from build123d import *

# Parameters (mm, degrees)
BOSS_EXTRUDE1_DEPTH = 4
BOSS_EXTRUDE2_DEPTH = 2.5
CHAMFER1_SIZE       = 1
SKETCH4_W           = 6
SKETCH4_H           = 1.5
CUT_EXTRUDE1_DEPTH  = 2.0001
CHAMFER2_SIZE       = 1
SKETCH5_W           = 39.95
SKETCH5_H           = 3.0001
BOSS_EXTRUDE3_DEPTH = 7.1


with BuildPart() as part:
    # Sketch2 → Boss-Extrude1 (new body)
    with BuildSketch(Plane.XY):
        Polygon((-29.9999, -3.0001), (29.9999, -3.0001), (29.9999, -34.771531454), (23.171531454, -41.5999), (-23.171531454, -41.5999), (-29.9999, -34.771531454), align=None)
        Polygon((-28, -33.943145751), (-28, -5), (28, -5), (28, -33.943145751), (22.343145751, -39.6), (-22.343145751, -39.6), align=None, mode=Mode.SUBTRACT)
    extrude(amount=-BOSS_EXTRUDE1_DEPTH)

    # Sketch3 → Boss-Extrude2 (add)
    with BuildSketch(Plane.XY):
        Polygon((-32, 0), (32, 0), (32, -35.6), (24, -43.6), (-24, -43.6), (-32, -35.6), align=None)
    extrude(amount=BOSS_EXTRUDE2_DEPTH)

    # Chamfer1
    chamfer1_edges = [part.edges().sort_by_distance(p)[0] for p in [
        (-32, -17.8, 2.5),
        (-28, -39.6, 2.5),
        (0, -43.6, 2.5),
        (28, -39.6, 2.5),
        (32, -17.8, 2.5),
        (0, 0, 2.5),
    ]]
    chamfer(chamfer1_edges, length=CHAMFER1_SIZE)

    # Sketch4 → Cut-Extrude1 (cut)
    with BuildSketch(Plane.XZ.offset(43.6)):
        Rectangle(SKETCH4_W, SKETCH4_H)
    extrude(amount=-CUT_EXTRUDE1_DEPTH, mode=Mode.SUBTRACT)

    # Chamfer2
    # the kernel refuses this chamfer: 1 mm, written as the material it adds along each edge
    with BuildSketch(Plane(origin=(3, -43.6, 0.75), x_dir=(0.027495876610586487, 0, -0.9996219169112968), z_dir=(0, 1, 0))) as chamfer2_piece_1_section:
        Polygon((CHAMFER2_SIZE * 0.999621916911, CHAMFER2_SIZE * 0.0274958766106), (-CHAMFER2_SIZE * 0.0274958766106, CHAMFER2_SIZE * 0.999621916911), (0, 0), align=None)
    chamfer2_piece_1 = extrude(amount=4.571782988, mode=Mode.PRIVATE)
    chamfer2_piece_1 = split(chamfer2_piece_1, bisect_by=Plane(origin=(2.65, -42.59995, 0), z_dir=(0, 0, 1)), keep=Keep.TOP, mode=Mode.PRIVATE)
    add(chamfer2_piece_1)
    with BuildSketch(Plane(origin=(-3, -43.6, 0.75), x_dir=(-0.027495876610586487, 0, -0.9996219169112968), z_dir=(0, 1, 0))) as chamfer2_piece_2_section:
        Polygon((CHAMFER2_SIZE * 0.999621916911, -CHAMFER2_SIZE * 0.0274958766106), (-CHAMFER2_SIZE * 0.0274958766106, -CHAMFER2_SIZE * 0.999621916911), (0, 0), align=None)
    chamfer2_piece_2 = extrude(amount=4.571782988, mode=Mode.PRIVATE)
    chamfer2_piece_2 = split(chamfer2_piece_2, bisect_by=Plane(origin=(-2.65, -42.59995, 0), z_dir=(0, 0, 1)), keep=Keep.TOP, mode=Mode.PRIVATE)
    add(chamfer2_piece_2)

    # Sketch5 → Boss-Extrude3 (add)
    with BuildSketch(Plane(origin=(0, 0, 0), x_dir=(-1, 0, 0), z_dir=(0, 0, -1))):
        with Locations((0, -1.50005)):
            Rectangle(SKETCH5_W, SKETCH5_H)
    extrude(amount=BOSS_EXTRUDE3_DEPTH)


solid = part.part
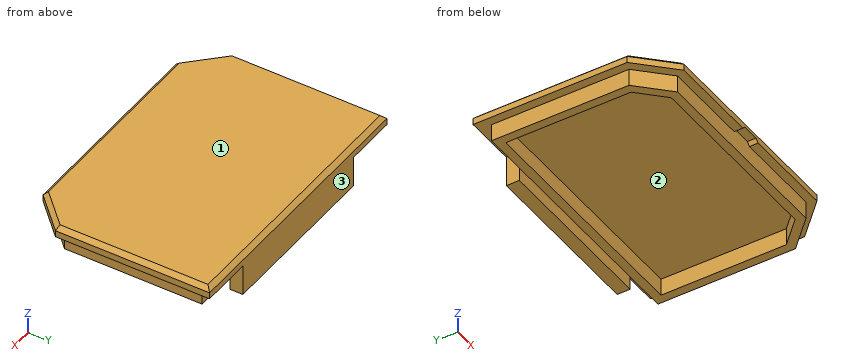
Geometry check sheet. Reference: the model listing, model coordinates, mm. Face numbers are marked on the shaded views. Coordinates: 2 decimals unless noted, no trailing zeros. Order: outer loops, then holes, each group sorted by start corner. A loop starts at its lowest first (then second) coordinate and runs counter-clockwise, first axis right, second up. Notation, with made-up numbers: (29, 45) - (80, 45) arc R6 cw to (80, 51) - close; hole circle Ø2 at (15, 33.5). An arc over 180 degrees is marked (long way). Answer in a Markdown table with one row per item. Add a question column.
1) Release check for a two-part mould opening along Y. For the marked faces 1, 2 and 3 record: +Y half, -Y half, draft (parallel to the pull), parting line (faces both ways), or undercut.
2) Cross-section at B-B, the plane x = 21.5. Record the cut outline in (y, z), then the cut area to 3 significant figures.
3) Gauge pin test, flat ends, axial feed: P1, Ø1.2, axis at x = -4, z = -2, coming from the -Y side; P2, Ø6, axis at x = 7.5, y = -31.5, coming from the -Z side; P3, Ø2, axis at y = -26, z = -1.5, coming from the -X side. Record the tip position at first contact, or that the pin passes through.
4) Cross-section at A-A, the plane y = -6.5. Record the cut outline in (x, z).
5) Material ranges on line 1 along X through (y, z) = (-19, -2); line 2 along Y through (x, z) = (-10, -3.75); line 3 along Z through (x, y) = (-26, -23.5), recorded low to high. Write a range as [from, to].
6) Cross-section at C-C, the plane z = -5.75. Record the cut outline in (x, y) (3 decimals), then the cut area to 3 significant figures.
Check result:
| question | item | result |
|---|---|---|
| 1 | face 1 | draft |
| 1 | face 2 | undercut |
| 1 | face 3 | +Y half |
| 2 | outline | (-43.6, 0) - (-41.6, 0) - (-41.6, -4) - (-39.6, -4) - (-39.6, 0) - (-5, 0) - (-5, -4) - (-3, -4) - (-3, 0) - (0, 0) - (0, 1.5) - (-1, 2.5) - (-42.6, 2.5) - (-43.6, 1.5) - close |
| 2 | area | 124 mm² |
| 3 | P1 | stops at y = -41.6 |
| 3 | P2 | stops at z = 0 |
| 3 | P3 | stops at x = -30 |
| 4 | outline | (-32, 0) - (-30, 0) - (-30, -4) - (-28, -4) - (-28, 0) - (28, 0) - (28, -4) - (30, -4) - (30, 0) - (32, 0) - (32, 1.5) - (31, 2.5) - (-31, 2.5) - (-32, 1.5) - close |
| 5 | line 1 | x = [-30, -28], [28, 30] |
| 5 | line 2 | y = [-41.6, -39.6], [-5, 0] |
| 5 | line 3 | z = [0, 2.5] |
| 6 | outline | (-19.975, -3) - (19.975, -3) - (19.975, 0) - (-19.975, 0) - close |
| 6 | area | 120 mm² |
